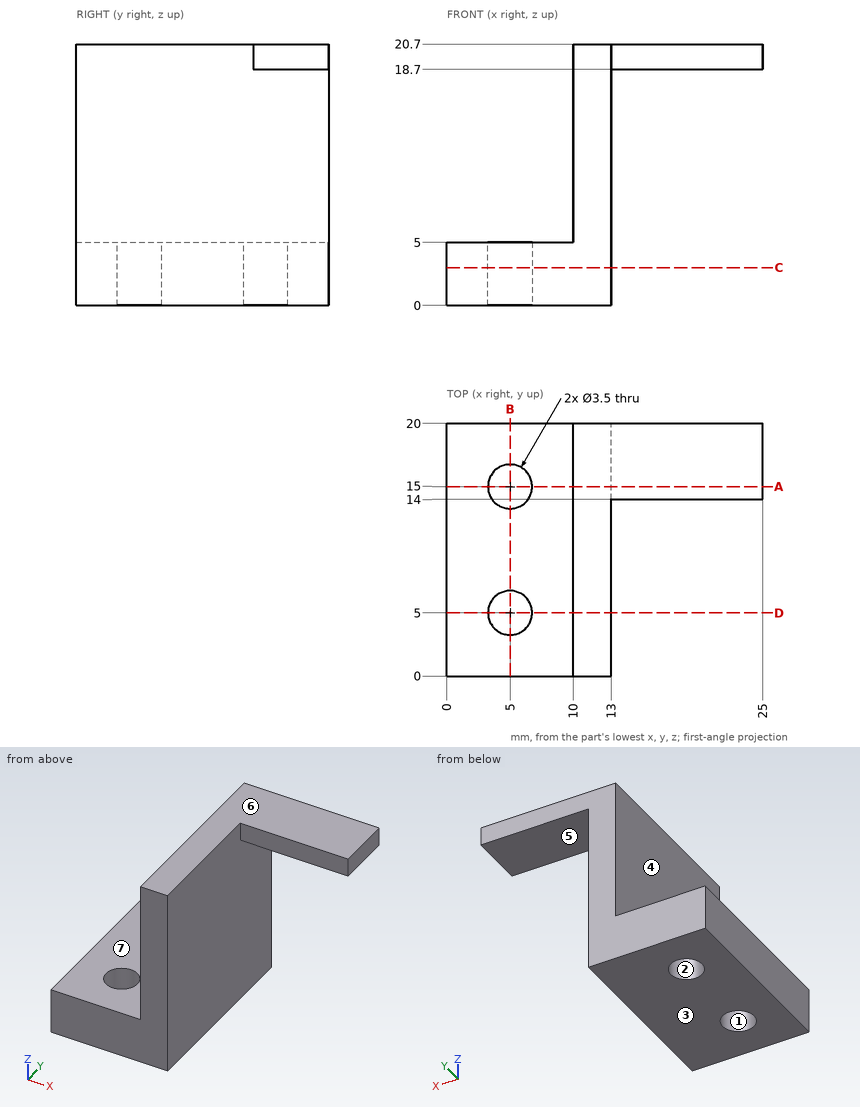
Geometry check sheet. Reference: drawing and pictorial views, mm from the part's lowest x, y, z. A direction names the side the tool comes from. Round coordinates to 2 decimals unless told otherwise and drop trailing zeros. Order: outer loops, then holes, each group sorted by start corner. A loop starts at its lowest first (then second) coordinate and runs counter-clockwise, first axis right, second up. Notation, with made-up numbers: (35.25, 88) - (88.25, 88) arc R29 ccw to (88.25, 112) - close; hole circle Ø1 at (-15, 19). An arc over 180 degrees is marked (long way). Use a Markdown table: item, result. Add a question column.
1) Mould release check, pull along X, two halves, no side actions. Record for the marked faces 1, 2, 3 and 4: released by +X, released by -X, zero draft, split by the parting line, or undercut.
2) Section check A-A (y = 15). Record the cut outline in (x, z).
3) Section check B-B (x = 5). Record the cut outline in (y, z).
4) Section check C-C (z = 3). Record the cut outline in (x, y), then the cut area to 3 significant figures.
5) Gauge pin test, flat ends, axial feed: P1, Ø6, axis at y = 11, z = 12, coming from the +X side; P2, Ø1.6, axis at x = 19.5, z = 19.5, coming from the -Y side; P3, Ø4.5, axis at y = 8.5, z = 12, coming from the -X side. Record the tip position at first contact, or that the pin passes through.
6) Set-up check for the marked faces 5, 6 and 7: record each of +Z, -Z, +X, -X, +Y, -Y from which the full face is reachable in a straight line by a thin tool's end or side.
7) Thickness scan on line 1 along Y through (x, z) = (5, 3.45); line 2 along X through (y, z) = (10, 19.25); line 3 along Y through (x, z) = (13.5, 19.5). Record the ranges inside material, lowest first.
8) Section check D-D (y = 5). Record the cut outline in (x, z), then the cut area to 3 significant figures.
Established:
| question | item | result |
|---|---|---|
| 1 | face 1 | undercut |
| 1 | face 2 | undercut |
| 1 | face 3 | zero draft |
| 1 | face 4 | released by -X |
| 2 | outline | (0, 0) - (3.25, 0) - (3.25, 5) - (0, 5) - close; (6.75, 0) - (13, 0) - (13, 18.7) - (25, 18.7) - (25, 20.7) - (10, 20.7) - (10, 5) - (6.75, 5) - close |
| 3 | outline | (0, 0) - (3.25, 0) - (3.25, 5) - (0, 5) - close; (6.75, 0) - (13.25, 0) - (13.25, 5) - (6.75, 5) - close; (16.75, 0) - (20, 0) - (20, 5) - (16.75, 5) - close |
| 4 | outline | (0, 0) - (13, 0) - (13, 20) - (0, 20) - close; hole circle Ø3.5 at (5, 5); hole circle Ø3.5 at (5, 15) |
| 4 | area | 241 mm2 |
| 5 | P1 | x = 13 |
| 5 | P2 | y = 14 |
| 5 | P3 | x = 10 |
| 6 | face 5 | -Z, +X, +Y, -Y |
| 6 | face 6 | +Z, +X, -X, +Y, -Y |
| 6 | face 7 | +Z, -X, +Y, -Y |
| 7 | line 1 | 0 to 3.25, 6.75 to 13.25, 16.75 to 20 |
| 7 | line 2 | 10 to 13 |
| 7 | line 3 | 14 to 20 |
| 8 | outline | (0, 0) - (3.25, 0) - (3.25, 5) - (0, 5) - close; (6.75, 0) - (13, 0) - (13, 20.7) - (10, 20.7) - (10, 5) - (6.75, 5) - close |
| 8 | area | 94.6 mm2 |
